Here's the drawing with two shaded views (mm, measured from the low corner). I have some questions. A direction names the side the tool comes from. Round coordinates to 2 decimals unless told otherwise and drop trailing zeros. Loops run counter-clockwise (first coordinate to the right, second up) from the corner with the lowest first, then second, coordinate; pieces in that order, holes last. Notation, with made-up numbers: (53.5, 0) - (101.5, 0) arc R24 ccw to (101.5, 31) - close; hole circle Ø9 at (65.25, -38.5). An arc over 180 degrees is marked (long way). Use one line per item in the form item = value.
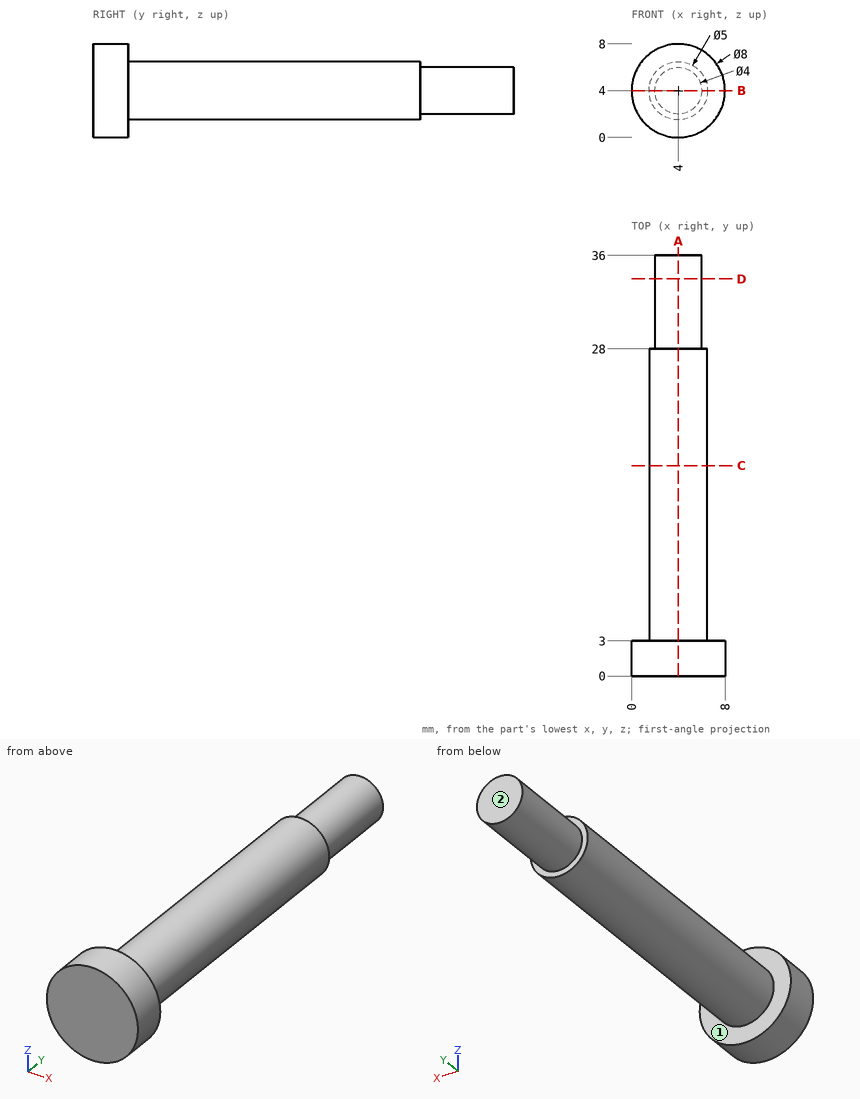
1. If we section it at C-C, the plane y = 18: Write out the boundary of the cut face in (x, z), plus the area to 3 significant figures.
Solution:
outline = circle Ø5 at (4, 4)
area = 19.6 mm^2
2. On a 3-axis mill with a long thin cutter (end or side, diameter ignored), from which of +Z, -Z, +X, -X, +Y, -Y can I reach the whole of each face in a straight line? I mean the marked faces 1 and 2. Say none if no direction works.
Solution:
face_1 = +Y
face_2 = +Z, -Z, +X, -X, +Y
3. If we section it at B-B, the plane z = 4: Write out the boundary of the cut face in (x, y).
Solution:
outline = (0, 0) - (8, 0) - (8, 3) - (6.5, 3) - (6.5, 28) - (6, 28) - (6, 36) - (2, 36) - (2, 28) - (1.5, 28) - (1.5, 3) - (0, 3) - close
4. If we section it at A-A, the plane x = 4: Write out the boundary of the cut face in (y, z).
Solution:
outline = (0, 0) - (3, 0) - (3, 1.5) - (28, 1.5) - (28, 2) - (36, 2) - (36, 6) - (28, 6) - (28, 6.5) - (3, 6.5) - (3, 8) - (0, 8) - close
5. If we section it at D-D, the plane y = 34: Write out the boundary of the cut face in (x, z), plus the area to 3 significant figures.
Solution:
outline = circle Ø4 at (4, 4)
area = 12.6 mm^2
6. For P1, Ø3, axis at y = 8, z = 1.5, coming from the -X side; P2, Ø1, axis at y = 19.5, z = 4.5, coming from the +X side, each with a flat end and sliding along its axis, tell me the tip position at first contact or that it passes through.
Solution:
P1 = 1.71
P2 = 6.5
7. Please list where these lines run through material, in increasing order: line 1 along Y through (x, z) = (7.25, 5); line 2 along Y through (x, z) = (5.75, 2.75); line 3 along X through (y, z) = (24, 5.5).
Solution:
line_1 = 0 to 3
line_2 = 0 to 28
line_3 = 2 to 6
